from build123d import *

# Parameters (mm, degrees)
F0_R     = 3.2
F1_DEPTH = 14
F2_R     = 7
F3_R     = 6.99999
F5_START = 5
F4_R     = 3.3
F5_DEPTH = 60
F7_START = -5
F6_R     = 3.3
F7_DEPTH = 60


# Not quite as in the source:
# - a fillet or chamfer is up to 0.001 mm smaller than in the source, because OpenCascade refuses the exact size


with BuildPart() as f1:
    # F0 (on Top) → F1 (new body)
    with BuildSketch(Plane.XY):
        with BuildLine():
            ThreePointArc((0, 58), (-5.6568542495, 55.6568542495), (-8, 50))
            Line((-8, 50), (-8, 38))
            ThreePointArc((-8, 38), (-16.7867965644, 16.7867965644), (-38, 8))
            Line((-38, 8), (-50, 8))
            ThreePointArc((-50, 8), (-55.6568542495, 5.6568542495), (-58, 0))
            ThreePointArc((-58, 0), (-55.6568542495, -5.6568542495), (-50, -8))
            Line((-50, -8), (-38, -8))
            ThreePointArc((-38, -8), (-16.7867965644, -16.7867965644), (-8, -38))
            Line((-8, -38), (-8, -50))
            ThreePointArc((-8, -50), (-5.6568542495, -55.6568542495), (0, -58))
            ThreePointArc((0, -58), (5.6568542495, -55.6568542495), (8, -50))
            Line((8, -50), (8, -38))
            ThreePointArc((8, -38), (16.7867965644, -16.7867965644), (38, -8))
            Line((38, -8), (50, -8))
            ThreePointArc((50, -8), (55.6568542495, -5.6568542495), (58, 0))
            ThreePointArc((58, 0), (55.6568542495, 5.6568542495), (50, 8))
            Line((50, 8), (38, 8))
            ThreePointArc((38, 8), (16.7867965644, 16.7867965644), (8, 38))
            Line((8, 38), (8, 50))
            ThreePointArc((8, 50), (5.6568542495, 55.6568542495), (0, 58))
        make_face()
        Circle(F0_R, mode=Mode.SUBTRACT)
    extrude(amount=F1_DEPTH)

    # F2
    f2_edges = [f1.edges().sort_by_distance(p)[0] for p in [
        (-16.786797, 16.786797, 14),
    ]]
    fillet(f2_edges, radius=F2_R)

    # F3 (radius 7 in the source; OpenCascade refuses exactly that, so slightly less here)
    f3_edges = [f1.edges().sort_by_distance(p)[0] for p in [
        (16.786797, 16.786797, 0),
    ]]
    fillet(f3_edges, radius=F3_R)

    # F4 (on Front) → F5 (cut)
    with BuildSketch(Plane.XZ.offset(F5_START)):
        with Locations((0, 7)):
            Circle(F4_R)
    extrude(amount=F5_DEPTH, mode=Mode.SUBTRACT)

    # F6 (on Right) → F7 (cut)
    with BuildSketch(Plane.YZ.offset(F7_START)):
        with Locations((0, 7)):
            Circle(F6_R)
    extrude(amount=-F7_DEPTH, mode=Mode.SUBTRACT)


solid = f1.part
Build history of the part. All positions in model axes, mm. A direction names the side the tool comes from. Give positions to 0.01 mm unless a question says otherwise; leave off trailing zeros. Use one line per item in the form item = value.
1) Drop flat-ended pins along their axis: pin 1 (3.5 mm diameter, centred on y = -0.5, z = 6, fed in from -X); pin 2 (3.5 mm diameter, centred on x = 1, z = 6, fed in from -Y); pin 3 (3 mm diameter, centred on x = -19.5, z = 8.5, fed in from +Y). Give the stop position or say it passes through.
Calculated:
pin_1 = -5
pin_2 = -5
pin_3 = 15.48
2) Probe probe 1 along Y at (x, z) = (-39, 6.75); probe 2 along Z at (x, y) = (0, -17); probe 3 along X at (y, z) = (-15.5, 9). List the from-to ranges inside material, lowest first.
Calculated:
probe_1 = -8 to -3.29, 3.29 to 8
probe_2 = 0 to 3.7, 10.3 to 14
probe_3 = -17.72 to -2.62, 2.62 to 17.72
3) Tool access for faces 1 (the face through (43.9, 6, 11.9)), 2 (the face through (-5.9, -44.1, 2)), 3 (the face through (-43.9, -6, 11.9)), 4 (the face through (-5.9, 43.9, 2)), 5 (the face through (-0.43, -30.78, 10.27)): list every direction of +Z, -Z, +X, -X, +Y, -Y with a clear straight run to the whole face (end or side of a thin tool).
Calculated:
face_1 = +Z, +X, +Y
face_2 = -Z, -X, -Y
face_3 = +Z, -X, -Y
face_4 = -Z, -X, +Y
face_5 = -Y
4) Two-plate mould, pull along Y, no slides. Class faces 6 (the face through (44.1, -6, 11.9)), 7 (the face through (-44.1, 6, 11.9)), 8 (the face through (-2.539, -1.947, 6.902)): released by +Y, released by -Y, zero draft, split by the parting line, or undercut.
Calculated:
face_6 = released by -Y
face_7 = released by +Y
face_8 = undercut
